Autodesk Inventor part; units mm, degrees
ref_plane "YZ Plane" through (0, 0, 0) normal (1, 0, 0) x (0, 1, 0)
ref_plane "XZ Plane" through (0, 0, 0) normal (0, 1, 0) x (-1, 0, 0)
ref_plane "XY Plane" through (0, 0, 0) normal (0, 0, 1) x (1, 0, 0)
sketch "Sketch1" plane through (0, 0, 0) normal (0, 0, 1) x (1, 0, 0)
  circle A0 centre (0, 0) radius 20
  dimension "d0" = 40
extrude "Extrusion1" add sketch "Sketch1" along normal blind 10
sketch "Sketch2" plane through (0, 0, 0) normal (0, 0, -1) x (-1, 0, 0)
  circle A0 centre (0, 0) radius 20
  line L0 (0, 0) -> (13.0166, -8.0397)
  line L1 (0, 0) -> (11.1647, -10.798)
  arc A1 (11.1647, -10.798) -> (13.0166, -8.0397) centre (12.1431, -9.454) ccw
extrude "Extrusion2" add sketch "Sketch2" along normal blind 1.5 contours L0 A1 L1
properties part number "hotbuton"
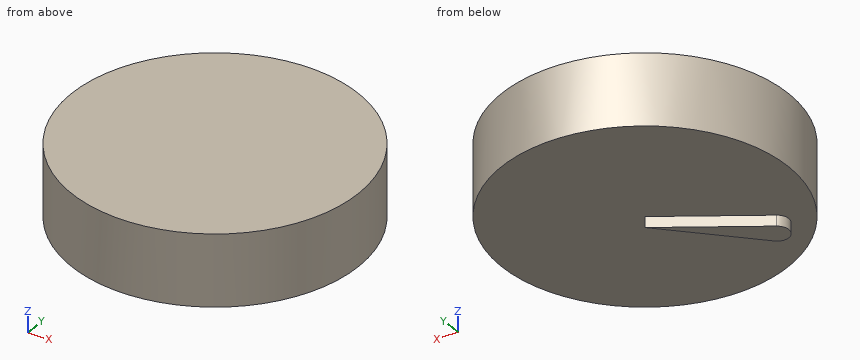
The model under review builds one solid part; all positions refer to its coordinate system, in mm. Give positions to 0.01 mm unless a question says otherwise; leave off trailing zeros. Write each loop counter-clockwise with the first axis right and the second up, starting at its lowest first coordinate (ties: lowest second). Pieces come first, ordered by that corner, then holes. Notation, with made-up numbers: M 2.25,-9.75 L 18.25,-9.75 A32 ccw 18.25,20.25 Z; hole C 33,19.5 d2. An arc over 180 degrees is marked long. Write each question's results on one line, items separated by ' | '. Start each with the question number.
1. We need section B-B (z = 2.75). Write out the cut boundary in (x, y), and give its area (3 significant figures).
2. Insertion check: pin 1 Ø2 at (x, z) = (4.5, 1) entering from +Y; pin 2 Ø5 at (y, z) = (1, 8.5) entering from -X; pin 3 Ø3 at (x, z) = (-5.5, 7) entering from +Y; pin 4 Ø2 at (x, y) = (-12, 2.5) entering from -Z. Each pin has a flat end and moves straight along its axis. Give the tip position at first contact, or say it passes through.
3. For probe 1 along Z at (x, y) = (1.5, 0); probe 2 along X at (y, z) = (0.5, 4.25); probe 3 along X at (y, z) = (3, 7.5), list the stretches that pass through material, from the lowest coordinate up. Write a range as [from, to].
4. We need section A-A (y = -3). Write out the cut boundary in (x, z).
5. We need section C-C (x = -4.5). Write out the cut boundary in (y, z).
6. We need section D-D (y = 15). Write out the cut boundary in (x, z).
Results found:
1) outline: C 0,0 d40 | area: 1,260 mm^2
2) pin 1: stops at y = 19.69 | pin 2: stops at x = -20 | pin 3: stops at y = 19.6 | pin 4: stops at z = 0
3) probe 1: z = [0, 10] | probe 2: x = [-19.99, 19.99] | probe 3: x = [-19.77, 19.77]
4) outline: M -19.77,0 L -4.86,0 L -4.86,-1.5 L -3.1,-1.5 L -3.1,0 L 19.77,0 L 19.77,10 L -19.77,10 Z
5) outline: M -19.49,0 L -4.35,0 L -4.35,-1.5 L -2.78,-1.5 L -2.78,0 L 19.49,0 L 19.49,10 L -19.49,10 Z
6) outline: M -13.23,0 L 13.23,0 L 13.23,10 L -13.23,10 Z
